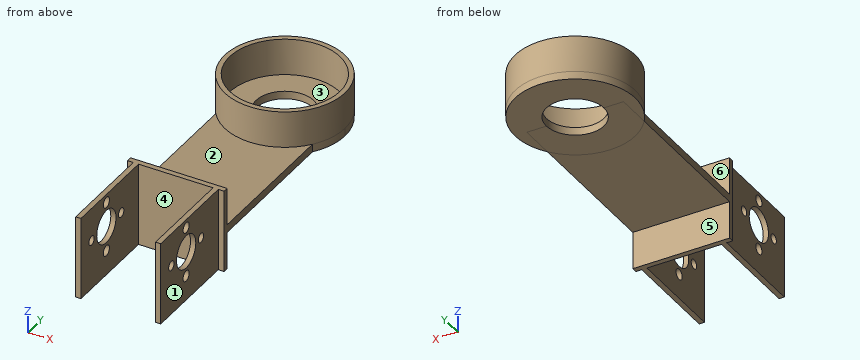
from build123d import *

# Parameters (mm, degrees)
SKETCH1_W                = 2
SKETCH1_H                = 31.74
BOSS_EXTRUDE1_DEPTH      = 40
BOSS_EXTRUDE1_2_DEPTH    = 40
SKETCH2_W                = 37
SKETCH2_H                = 31.74
BOSS_EXTRUDE3_DEPTH      = 2
SKETCH8_W                = 37
SKETCH8_H                = 3
BOSS_EXTRUDE4_DEPTH      = 70
SKETCH20_R               = 6.36
SKETCH20_R_2             = 1.78
SKETCH20_R_3             = 2.03
CUT_EXTRUDE4_DEPTH       = 3.24
CUT_EXTRUDE4_DEPTH_BACK  = 35.76
SKETCH23_R               = 23
BOSS_EXTRUDE6_DEPTH      = 14
BOSS_EXTRUDE6_DEPTH_BACK = 3
SKETCH25_R               = 21.1
CUT_EXTRUDE5_DEPTH       = 14
SKETCH26_R               = 11
CUT_EXTRUDE6_DEPTH       = 15.37
CUT_EXTRUDE6_DEPTH_BACK  = 18.37


with BuildPart() as part:
    # Sketch1 → Boss-Extrude1 (new body)
    with BuildSketch(Plane(origin=(0, 0, 0), x_dir=(1, 0, 0), z_dir=(0, 1, 0))):
        with Locations((-2.074327578, -14.662349727)):
            Rectangle(SKETCH1_W, SKETCH1_H)
    extrude(amount=BOSS_EXTRUDE1_DEPTH)



with BuildPart() as body_2:
    # Sketch1 → Boss-Extrude1 2 (new body)
    with BuildSketch(Plane(origin=(0, 0, 0), x_dir=(1, 0, 0), z_dir=(0, 1, 0))):
        with Locations((28.453672422, -14.662349727)):
            Rectangle(SKETCH1_W, SKETCH1_H)
    extrude(amount=BOSS_EXTRUDE1_2_DEPTH)


with BuildPart() as part_1:
    add(part.part)

    add(body_2.part)  # Boss-Extrude3 merges body 2
    # Sketch2 → Boss-Extrude3 (add)
    with BuildSketch(Plane(origin=(0, 40, 0), x_dir=(1, 0, 0), z_dir=(0, 1, 0))):
        with Locations((13.193672422, -14.662349727)):
            Rectangle(SKETCH2_W, SKETCH2_H)
    extrude(amount=-BOSS_EXTRUDE3_DEPTH)

    # Sketch8 → Boss-Extrude4 (add)
    with BuildSketch(Plane(origin=(0, 40, 0), x_dir=(1, 0, 0), z_dir=(0, 1, 0))):
        with Locations((13.193672422, -14.662349727)):
            Rectangle(SKETCH8_W, SKETCH8_H)
    extrude(amount=BOSS_EXTRUDE4_DEPTH)

    # Sketch20 → Cut-Extrude4 (cut, two sides)
    with BuildSketch(Plane(origin=(29.453672422, 0, 0), x_dir=(0, 0, -1), z_dir=(1, 0, 0))) as cut_extrude4_sk:
        with Locations((-17.842349727, 16.779878139)):
            Circle(SKETCH20_R)
        with Locations((-17.842349727, 26.558878139)):
            Circle(SKETCH20_R_2)
        with Locations((-17.842349727, 7.000878139)):
            Circle(SKETCH20_R_2)
        with Locations((-27.367349727, 16.779878139)):
            Circle(SKETCH20_R_3)
        with Locations((-8.317349727, 16.779878139)):
            Circle(SKETCH20_R_3)
    extrude(amount=CUT_EXTRUDE4_DEPTH, mode=Mode.SUBTRACT)
    extrude(cut_extrude4_sk.sketch, amount=-CUT_EXTRUDE4_DEPTH_BACK, mode=Mode.SUBTRACT)

    # Sketch23 → Boss-Extrude6 (add, two sides)
    with BuildSketch(Plane.XY.offset(16.162349727)) as boss_extrude6_sk:
        with Locations((13.193672422, 110)):
            Circle(SKETCH23_R)
    extrude(amount=BOSS_EXTRUDE6_DEPTH)
    extrude(boss_extrude6_sk.sketch, amount=-BOSS_EXTRUDE6_DEPTH_BACK)

    # Sketch25 → Cut-Extrude5 (cut)
    with BuildSketch(Plane.XY.offset(30.162349727)):
        with Locations((13.193672422, 110)):
            Circle(SKETCH25_R)
    extrude(amount=-CUT_EXTRUDE5_DEPTH, mode=Mode.SUBTRACT)

    # Sketch26 → Cut-Extrude6 (cut, two sides)
    with BuildSketch(Plane.XY.offset(16.162349727)) as cut_extrude6_sk:
        with Locations((13.193672422, 110)):
            Circle(SKETCH26_R)
    extrude(amount=CUT_EXTRUDE6_DEPTH, mode=Mode.SUBTRACT)
    extrude(cut_extrude6_sk.sketch, amount=-CUT_EXTRUDE6_DEPTH_BACK, mode=Mode.SUBTRACT)


solid = part_1.part
Verification items for the finished model (mm, model axes). Face numbers are marked on the shaded views. A direction names the side the tool comes from. Round coordinates to 2 decimals unless told otherwise and drop trailing zeros. Loops run counter-clockwise (first coordinate to the right, second up) from the corner with the lowest first, then second, coordinate; pieces in that order, holes last. Notation, with made-up numbers: (-6, 80.25) - (36, 80.25) arc R25 cw to (36, 103.25) - close; hole circle Ø5 at (82, -16.75). An arc over 180 degrees is marked (long way). Use a Markdown table: item, result. Add a question column.
1. Access from +Z, -Z, +X, -X, +Y, -Y to the whole of each face (thin tool, end or side, straight path). Record for the marked faces 4, 5 and 6.
2. Section check D-D, the plane z = 9. Record the boundary of the cut face in (x, y).
3. Section check A-A, the plane z = 1. Record the boundary of the cut face in (x, y), plus the area to 3 significant figures.
4. Gauge pin test, flat ends, axial feed: pin 1 (16 mm diameter, centred on y = 65.5, z = 8, fed in from -X); pin 2 (7 mm diameter, centred on x = 7, z = 6, fed in from +Y); pin 3 (12 mm diameter, centred on x = 5, z = 22.5, fed in from -Y). Record the tip position at first contact, or that the pin passes through.
5. Release check for a two-part mould opening along X. For the marked faces 1, 2 and 3 record: released by +X, released by -X, zero draft, split by the parting line, or undercut.
6. Section check C-C, the plane x = 19.5. Record the boundary of the cut face in (y, z).
7. Section check B-B, the plane y = 21.5. Record the boundary of the cut face in (x, z), plus the area to 3 significant figures.
8. Thickness scan on probe 1 along Y at (x, z) = (19, 24); probe 2 along Y at (x, z) = (-2, 20); probe 3 along Z at (x, y) = (26.5, 126). Record the ranges inside material, lowest first. Write a range as [from, to].
Checks:
| question | item | result |
|---|---|---|
| 1 | face 4 | +Z, -Z, -Y |
| 1 | face 5 | -Z, +X, -X, +Y |
| 1 | face 6 | +Z, +X, -X |
| 2 | outline | (-5.31, 38) - (-3.07, 38) - (-3.07, 18.69) - (-1.07, 18.69) - (-1.07, 38) - (27.45, 38) - (27.45, 18.69) - (29.45, 18.69) - (29.45, 38) - (31.69, 38) - (31.69, 40) - (-5.31, 40) - close; (-3.07, 0) - (-1.07, 0) - (-1.07, 14.87) - (-3.07, 14.87) - close; (27.45, 0) - (29.45, 0) - (29.45, 14.87) - (27.45, 14.87) - close |
| 3 | outline | (-5.31, 38) - (-3.07, 38) - (-3.07, 0) - (-1.07, 0) - (-1.07, 38) - (27.45, 38) - (27.45, 0) - (29.45, 0) - (29.45, 38) - (31.69, 38) - (31.69, 40) - (-5.31, 40) - close |
| 3 | area | 226 mm^2 |
| 4 | pin 1 | stops at x = -5.31 |
| 4 | pin 2 | stops at y = 40 |
| 4 | pin 3 | stops at y = 38 |
| 5 | face 1 | released by +X |
| 5 | face 2 | zero draft |
| 5 | face 3 | undercut |
| 6 | outline | (38, -1.21) - (40, -1.21) - (40, 13.16) - (100.99, 13.16) - (100.99, 16.16) - (89.86, 16.16) - (89.86, 30.16) - (87.88, 30.16) - (87.88, 16.16) - (40, 16.16) - (40, 30.53) - (38, 30.53) - close; (119.01, 13.16) - (132.12, 13.16) - (132.12, 30.16) - (130.14, 30.16) - (130.14, 16.16) - (119.01, 16.16) - close |
| 7 | outline | (-3.07, -1.21) - (-1.07, -1.21) - (-1.07, 13.58) - (-3.07, 13.58) - close; (-3.07, 22.1) - (-1.07, 22.1) - (-1.07, 30.53) - (-3.07, 30.53) - close; (27.45, -1.21) - (29.45, -1.21) - (29.45, 13.58) - (27.45, 13.58) - close; (27.45, 22.1) - (29.45, 22.1) - (29.45, 30.53) - (27.45, 30.53) - close |
| 7 | area | 92.9 mm^2 |
| 8 | probe 1 | y = [38, 40], [87.74, 89.71], [130.29, 132.26] |
| 8 | probe 2 | y = [0, 10.8], [22.76, 40], [92.73, 95.36], [124.64, 127.27] |
| 8 | probe 3 | z = [13.16, 16.16] |
